The listing builds one solid part. Answer for the finished solid, in the listing's coordinates (mm). A direction names the side the tool comes from. Round coordinates to 2 decimals unless told otherwise and drop trailing zeros. Write each loop counter-clockwise with the first axis right and the second up, starting at its lowest first coordinate (ties: lowest second). Pieces come first, ordered by that corner, then holes. Notation, with made-up numbers: (74, 43.5) - (131, 43.5) arc R26 cw to (131, 63.5) - close; hole circle Ø7 at (-23, -31.75). An arc over 180 degrees is marked (long way). Return JSON: item names as keys, results as strings. Group by question number.
(1) Section B-B, the plane x = 0 is taken. Write down the section's boundary in (y, z), then the cut area to 3 significant figures.
(2) Section A-A, the plane y = 0 is taken. Write down the section's boundary in (x, z).
(3) Determine the mould class of faces 4 (the cylindrical face through (27.14, -13.345, -9.079)), 5 (the conical face through (-22.717, -12.417, -10.201)), 6 (the flat face through (-30.838, 0, -10)), 7 (the flat face through (0, 17.5, -10)) for opening direction Y: +Y half, -Y half, draft (parallel to the pull), parting line (faces both ways), or undercut.
(4) Which of the six approach directions +Z, -Z, +X, -X, +Y, -Y give full straight-line access (tool end or side, diameter ignored) to faces 1 (the flat face through (30.838, 0, -10)), 2 (the cylindrical face through (-27.14, 11.655, -9.079)), 3 (the cylindrical face through (27.14, 11.655, -9.079))?
(5) Find the intervals of material crossed by line 1 along Y through (x, z) = (-25.25, -10); line 2 along Z through (x, y) = (-24.75, -12.5); line 3 along Y through (x, z) = (28, -11), in increasing order. Write a range as [from, to].
(6) Each of these flat-tipped pins is pushed along its axis until it touches: pin 1 (2 mm diameter, centred on y = -12.5, z = -10, fed in from +X); pin 2 (3 mm diameter, centred on y = 12.5, z = -10, fed in from +X). Where does it stop, or does it pass through?
```python
from build123d import *

# Parameters (mm, degrees)
SKETCH2_W                            = 61.675
SKETCH2_H                            = 35
BOSS_EXTRUDE1_DEPTH                  = 20
TAP_DRILL_FOR_M6X1_0_TAP1_D          = 5
TAP_DRILL_FOR_M3X0_5_TAP1_AT_2_COUNT = 2
TAP_DRILL_FOR_M3X0_5_TAP1_AT_2_PITCH = 25
FILLET1_R                            = 1


with BuildPart() as part:
    # Sketch2 → Boss-Extrude1 (new body)
    with BuildSketch(Plane.XY):
        Rectangle(SKETCH2_W, SKETCH2_H)
    extrude(amount=-BOSS_EXTRUDE1_DEPTH)

    # Tap Drill for M6x1.0 Tap1 (through all)
    with Locations(Plane.XY):
        with Locations((0, 0)):
            Hole(TAP_DRILL_FOR_M6X1_0_TAP1_D / 2)

    # Sketch6 → Tap Drill for M3x0.5 Tap1 (revolve, cut)
    with BuildSketch(Plane(origin=(30.8375, 12.5, -10), x_dir=(0, 0, -1), z_dir=(0, 1, 0))):
        Polygon((0, 0), (0, 8.251075774), (1.25, 7.5), (1.25, 0), align=None)
    tap_drill_for_m3x0_5_tap1 = revolve(axis=Axis((37.1875, 12.5, -10), (-1, 0, 0)), mode=Mode.SUBTRACT)

    # Tap Drill for M3x0.5 Tap1 at 2: Tap Drill for M3x0.5 Tap1 ×2
    with Locations(*[(0, -i * TAP_DRILL_FOR_M3X0_5_TAP1_AT_2_PITCH, 0) for i in range(1, TAP_DRILL_FOR_M3X0_5_TAP1_AT_2_COUNT)]):
        add(tap_drill_for_m3x0_5_tap1, mode=Mode.SUBTRACT)

    # Mirror1: Tap Drill for M3x0.5 Tap1 across plane
    add(tap_drill_for_m3x0_5_tap1.mirror(Plane(origin=(0, 0, 0), x_dir=(0, 0, 1), z_dir=(1, 0, 0))), mode=Mode.SUBTRACT)

    # Mirror1 copy 1 sketch → Mirror1 copy 1 (revolve, cut)
    with BuildSketch(Plane(origin=(-30.8375, -12.5, -10), x_dir=(0, 0, -1), z_dir=(0, 1, 0))):
        Polygon((0, 0), (0, -8.251075774), (1.25, -7.5), (1.25, 0), align=None)
    revolve(axis=Axis((-37.1875, -12.5, -10), (-1, 0, 0)), mode=Mode.SUBTRACT)

    # Fillet1
    fillet1_edges = [part.edges().sort_by_distance(p)[0] for p in [
        (0, 17.5, 0),
        (0, -17.5, 0),
    ]]
    fillet(fillet1_edges, radius=FILLET1_R)


solid = part.part
```
Working result:
{
 "1": {"outline": "(-17.5, -20) - (-2.5, -20) - (-2.5, 0) - (-16.5, 0) arc R1 ccw to (-17.5, -1) - close; (2.5, -20) - (17.5, -20) - (17.5, -1) arc R1 ccw to (16.5, 0) - (2.5, 0) - close", "area": "600 mm^2"},
 "2": {"outline": "(-30.84, -20) - (-2.5, -20) - (-2.5, 0) - (-30.84, 0) - close; (2.5, -20) - (30.84, -20) - (30.84, 0) - (2.5, 0) - close"},
 "3": {"face 4": "undercut", "face 5": "undercut", "face 6": "draft", "face 7": "+Y half"},
 "4": {"face 1": "+Z, -Z, +X, +Y, -Y", "face 2": "-X", "face 3": "+X"},
 "5": {"line 1": "y = [-17.5, -13.75], [-11.25, 11.25], [13.75, 17.5]", "line 2": "z = [-20, -11.25], [-8.75, 0]", "line 3": "y = [-17.5, -13.25], [-11.75, 11.75], [13.25, 17.5]"},
 "6": {"pin 1": "stops at x = 23.19", "pin 2": "stops at x = 30.84"}
}
